Verification items for the finished model (mm, model axes). Face numbers are marked on the shaded views. A direction names the side the tool comes from. Coordinates: 2 decimals unless noted, no trailing zeros. Write each loop counter-clockwise with the first axis right and the second up, starting at its lowest first coordinate (ties: lowest second). Pieces come first, ordered by that corner, then holes. Notation, with made-up numbers: (-30, 16) -> (8, 16) arc R33 ccw to (8, 45) -> close; hole circle Ø5 at (63, 8). An arc over 180 degrees is marked (long way). Answer in a Markdown table with one row per item.
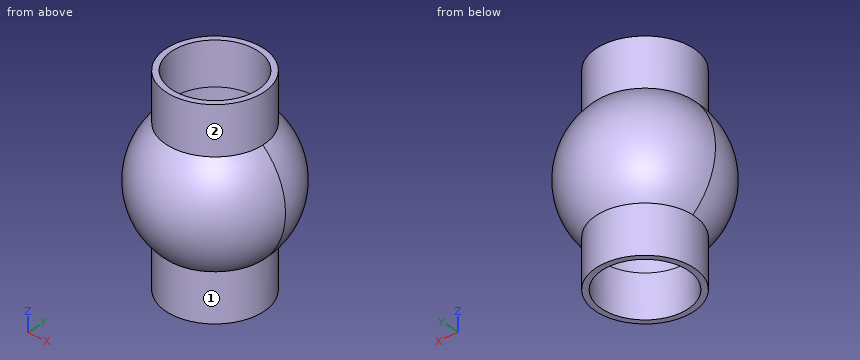
```python
from build123d import *

# Parameters (mm, degrees)
SKETCH2_R               = 1.5
CUT_EXTRUDE1_DEPTH      = 3.5
CUT_EXTRUDE1_DEPTH_BACK = 3.5
SKETCH2_3_R             = 1.7
SKETCH2_3_R_2           = 1.5
BOSS_EXTRUDE1_DEPTH     = 3.5


with BuildPart() as part:
    # Sketch1 one side → Revolve1 (revolve)
    with BuildSketch(Plane.XY):
        with BuildLine():
            ThreePointArc((0, -2.5), (1.767766953, -1.767766953), (2.5, 0))
            ThreePointArc((2.5, 0), (1.767766953, 1.767766953), (0, 2.5))
            Line((0, 2.5), (0, -2.5))
        make_face()
    revolve(axis=Axis((0, 2.75, 0), (0, -1, 0)))

    # Sketch2 → Cut-Extrude1 (cut, two sides)
    with BuildSketch(Plane.XY) as cut_extrude1_sk:
        Circle(SKETCH2_R)
    extrude(amount=CUT_EXTRUDE1_DEPTH, mode=Mode.SUBTRACT)
    extrude(cut_extrude1_sk.sketch, amount=-CUT_EXTRUDE1_DEPTH_BACK, mode=Mode.SUBTRACT)

    # Sketch2<3> → Boss-Extrude1 (add, symmetric)
    with BuildSketch(Plane.XY):
        Circle(SKETCH2_3_R)
        Circle(SKETCH2_3_R_2, mode=Mode.SUBTRACT)
    extrude(amount=BOSS_EXTRUDE1_DEPTH, both=True)


solid = part.part
```
1. Depth check by flat-ended pin: P1, Ø1.5, axis at y = 1.5, z = 1.5, coming from the -X side; P2, Ø1.5, axis at y = -1.5, z = 2.5, coming from the -X side. Enter the tip coordinate at first touch or a pass-through.
Geometry says:
| item | result |
|---|---|
| P1 | x = -2.09 |
| P2 | x = -1.53 |
2. Tool access check on the marked faces 1 and 2. Record the directions out of +Z, -Z, +X, -X, +Y, -Y that give a thin tool (end or side, any length) a straight path to the whole face; none if there is none.
Geometry says:
| item | result |
|---|---|
| face 1 | -Z |
| face 2 | +Z |
3. Thickness scan on line 1 (Y direction, x = 0, z = 2.9); line 2 (X direction, y = 0, z = 0). Record the ranges inside material, lowest first. Write a range as from..to.
Geometry says:
| item | result |
|---|---|
| line 1 | -1.7..-1.5, 1.5..1.7 |
| line 2 | -2.5..-1.5, 1.5..2.5 |
4. Section check B-B, the plane y = -0.2. Record the boundary of the cut face in (x, z).
Geometry says:
| item | result |
|---|---|
| outline | (-1.69, -3.5) -> (-1.49, -3.5) -> (-1.49, 3.5) -> (-1.69, 3.5) -> (-1.69, 1.83) arc R2.49 ccw to (-1.69, -1.83) -> close; (1.49, -3.5) -> (1.69, -3.5) -> (1.69, -1.83) arc R2.49 ccw to (1.69, 1.83) -> (1.69, 3.5) -> (1.49, 3.5) -> close |
5. Section check C-C, the plane z = 2.5. Record the boundary of the cut face in (x, y).
Geometry says:
| item | result |
|---|---|
| outline | circle Ø3.4 at (0, 0); hole circle Ø3 at (0, 0) |
6. Section check A-A, the plane x = 0. Record the boundary of the cut face in (y, z).
Geometry says:
| item | result |
|---|---|
| outline | (-1.7, -3.5) -> (-1.5, -3.5) -> (-1.5, 3.5) -> (-1.7, 3.5) -> (-1.7, 1.83) arc R2.5 ccw to (-1.7, -1.83) -> close; (1.5, -3.5) -> (1.7, -3.5) -> (1.7, -1.83) arc R2.5 ccw to (1.7, 1.83) -> (1.7, 3.5) -> (1.5, 3.5) -> close |
7. Section check D-D, the plane z = 1. Record the boundary of the cut face in (x, y), plus the area to 3 significant figures.
Geometry says:
| item | result |
|---|---|
| outline | circle Ø4.58 at (0, 0); hole circle Ø3 at (0, 0) |
| area | 9.42 mm^2 |
